Geometry: final body of the model. Coordinates: model frame, mm. Face numbers are marked on the shaded views. A direction names the side the tool comes from. Give positions to 0.01 mm unless a question says otherwise; leave off trailing zeros. Write each loop counter-clockwise with the first axis right and the second up, starting at its lowest first coordinate (ties: lowest second). Pieces come first, ordered by that corner, then holes. Notation, with made-up numbers: (16.5, 69) -> (43.5, 69) arc R35 ccw to (43.5, 102) -> close; hole circle Ø8 at (35, 16). An arc over 180 degrees is marked (long way). Answer in a Markdown table with one row per item. Add a question column.
Item 1: Section query B-B on z = 13.75. Output: boundary loops of the cut face in (x, y) (3 decimals), plus the area to 3 significant figures.
Item 2: Section query D-D on x = -22.5. Output: boundary loops of the cut face in (y, z), plus the area to 3 significant figures.
Item 3: Section query C-C on x = -48. Output: boundary loops of the cut face in (y, z), plus the area to 3 significant figures.
Item 4: First-contact query: P1, Ø6, axis at x = -17, y = 24.5, coming from the -Z side; P2, Ø5, axis at x = -27, z = 7, coming from the +Y side; P3, Ø1, axis at y = 26.5, z = 13, coming from the -X side; P4, Ø1, axis at x = -27, z = 2.5, coming from the +Y side. Flat tips, straight axial feed; report the tip coordinate or a pass-through.
Item 5: Access query for the marked faces 1 and 2. Directions: +Z, -Z, +X, -X, +Y, -Y. A direction counts if a zero-diameter tool reaches every point of the face in a straight line with its end or side. Return the directions, or none.
Item 6: Draft query along Y for the marked faces 3, 4 and 5. Return one class per face: +Y half, -Y half, draft (parallel to the pull), parting line (faces both ways), or undercut.
Item 7: Section query A-A on y = 11. Output: boundary loops of the cut face in (x, z).
Item 8: Material intervals for probe 1 along Y at (x, z) = (-36, 19.5); probe 2 along X at (y, z) = (24.5, 7.25); probe 3 along Y at (x, z) = (-27, 2), sorted ascending. Write a range as from..to.
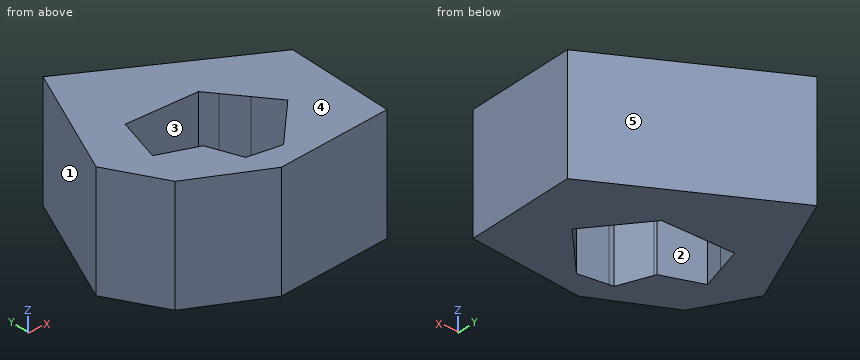
```python
from build123d import *

# Parameters (mm, degrees)
F1_DEPTH = 25.4


with BuildPart() as f1:
    # F0 (on Top) → F1 (new body)
    with BuildSketch(Plane.XY):
        Polygon((-49.4661442935, 49.9131269753), (-49.4661442935, 28.7559218705), (-45.0052889839, 28.7559218705), align=None)
        Polygon((-62.5776574016, 21.3062018156), (-49.4661442935, 28.7559218705), (-49.4661442935, 49.9131269753), align=None)
        Polygon((-51.2835987262, 22.9573797383), (-49.4661442935, 28.7559218705), (-62.5776574016, 21.3062018156), align=None)
        Polygon((-49.4661442935, 49.9131269753), (-45.0052889839, 28.7559218705), (-32.8907538248, 28.7559218705), align=None)
        Polygon((-52.9081679909, 17.7742328277), (-51.2835987262, 22.9573797383), (-62.5776574016, 21.3062018156), align=None)
        Polygon((-11.6215646267, 28.7559218705), (-49.4661442935, 49.9131269753), (-32.8907538248, 28.7559218705), align=None)
        Polygon((-52.9081679909, 17.7742328277), (-62.5776574016, 21.3062018156), (-55.7239130139, 8.7906699628), align=None)
        Polygon((-11.6215646267, 28.7559218705), (-32.8907538248, 28.7559218705), (-30.7049791526, 25.9659494027), align=None)
        Polygon((-44.056481693, 14.0725475488), (-44.2558990488, 14.6138233913), (-52.9081679909, 17.7742328277), (-55.7239130139, 8.7906699628), align=None)
        Polygon((-23.3790820657, 16.6150078645), (-11.6215646267, 28.7559218705), (-27.3222628842, 21.6481734783), align=None)
        Polygon((-12.8135187551, 3.1288827304), (-11.6215646267, 28.7559218705), (-23.3790820657, 16.6150078645), align=None)
        Polygon((-27.3222628842, 21.6481734783), (-11.6215646267, 28.7559218705), (-30.7049791526, 25.9659494027), align=None)
        Polygon((-41.4149532636, 6.9026825177), (-55.7239130139, 8.7906699628), (-39.0365384519, 0.4469832347), align=None)
        Polygon((-44.056481693, 14.0725475488), (-55.7239130139, 8.7906699628), (-41.4149532636, 6.9026825177), align=None)
        Polygon((-30.2658398726, 9.5036823021), (-12.8135187551, 3.1288827304), (-26.9007566578, 12.9784962793), align=None)
        Polygon((-39.0365384519, 0.4469832347), (-12.8135187551, 3.1288827304), (-33.7625144996, 5.8929858967), align=None)
        Polygon((-26.9007566578, 12.9784962793), (-12.8135187551, 3.1288827304), (-23.3790820657, 16.6150078645), align=None)
        Polygon((-33.7625144996, 5.8929858967), (-12.8135187551, 3.1288827304), (-30.2658398726, 9.5036823021), align=None)
        Polygon((-40.3685695275, 6.7646180189), (-39.0365384519, 0.4469832347), (-33.7625144996, 5.8929858967), align=None)
        Polygon((-41.4149532636, 6.9026825177), (-39.0365384519, 0.4469832347), (-40.3685695275, 6.7646180189), align=None)
    extrude(amount=F1_DEPTH)


solid = f1.part
```
Findings below:
| question | item | result |
|---|---|---|
| 1 | outline | (-62.578, 21.306) -> (-55.724, 8.791) -> (-39.037, 0.447) -> (-12.814, 3.129) -> (-11.622, 28.756) -> (-49.466, 49.913) -> close; hole (-52.908, 17.774) -> (-44.256, 14.614) -> (-41.415, 6.903) -> (-33.763, 5.893) -> (-23.379, 16.615) -> (-32.891, 28.756) -> (-49.466, 28.756) -> close |
| 1 | area | 1,270 mm^2 |
| 2 | outline | (2.14, 0) -> (34.84, 0) -> (34.84, 25.4) -> (2.14, 25.4) -> close |
| 2 | area | 831 mm^2 |
| 3 | outline | (4.93, 0) -> (15.98, 0) -> (15.98, 25.4) -> (4.93, 25.4) -> close; (28.76, 0) -> (49.09, 0) -> (49.09, 25.4) -> (28.76, 25.4) -> close |
| 3 | area | 797 mm^2 |
| 4 | P1 | stops at z = 0 |
| 4 | P2 | stops at y = 38.75 |
| 4 | P3 | stops at x = -60.43 |
| 4 | P4 | stops at y = 37.63 |
| 5 | face 1 | +Z, -Z, -X, +Y |
| 5 | face 2 | +Z, -Z |
| 6 | face 3 | undercut |
| 6 | face 4 | draft |
| 6 | face 5 | +Y half |
| 7 | outline | (-56.93, 0) -> (-42.92, 0) -> (-42.92, 25.4) -> (-56.93, 25.4) -> close; (-28.82, 0) -> (-12.45, 0) -> (-12.45, 25.4) -> (-28.82, 25.4) -> close |
| 8 | probe 1 | y = 0.76..6.19, 28.76..42.38 |
| 8 | probe 2 | x = -61.11..-50.8, -29.56..-11.82 |
| 8 | probe 3 | y = 1.68..12.88, 21.24..37.35 |
